Read the model definition and answer for the solid it produces. Units are mm, in the model's axes. Face numbers are marked on the shaded views. A direction names the side the tool comes from. Coordinates: 2 decimals unless noted, no trailing zeros. Loops run counter-clockwise (first coordinate to the right, second up) from the corner with the lowest first, then second, coordinate; pieces in that order, holes last. Notation, with made-up numbers: (-23, -12) -> (30, -12) arc R29 ccw to (30, 24) -> close; hole circle Ø9 at (62.25, -34). An arc over 180 degrees is marked (long way). Answer as CSV lines item,"result".
```python
from build123d import *

# Parameters (mm, degrees)
SKETCH_1_W          = 68.077724156
SKETCH_1_H          = 41.280670561
SKETCH_1_W_2        = 40
SKETCH_1_H_2        = 14
EXTRUDE_1_DEPTH     = 3
SKETCH_2_W          = 68.077724156
SKETCH_2_H          = 41.280670561
SKETCH_2_W_2        = 62.677724156
SKETCH_2_H_2        = 35.480670561
EXTRUDE_2_DEPTH     = 11.04005
SKETCH_3_W          = 7.040050383
SKETCH_3_H          = 11.280670561
CUT_EXTRUDE_1_DEPTH = 2.9
SKETCH_4_W          = 3
SKETCH_4_H          = 1.8
EXTRUDE_3_DEPTH     = 3
SKETCH_5_W          = 3
SKETCH_5_H          = 1.8
EXTRUDE_4_DEPTH     = 3
SKETCH_6_W          = 3
SKETCH_6_H          = 1.8
EXTRUDE_5_DEPTH     = 2
SKETCH_7_W          = 3
SKETCH_7_H          = 1.8
EXTRUDE_6_DEPTH     = 2
SKETCH_8_W          = 14
SKETCH_8_H          = 5
CUT_EXTRUDE_2_DEPTH = 2.9
SKETCH_9_W          = 1
SKETCH_9_H          = 15
CUT_EXTRUDE_3_DEPTH = 1
SKETCH_10_W         = 1.5
SKETCH_10_H         = 7
EXTRUDE_7_DEPTH     = 7
SKETCH_13_R         = 1.55
CUT_EXTRUDE_6_DEPTH = 2.5
SKETCH_14_W         = 4
SKETCH_14_H         = 1.5
EXTRUDE_8_DEPTH     = 11
SKETCH_15_W         = 4
SKETCH_15_H         = 1.5
EXTRUDE_9_DEPTH     = 10
CHAMFER_1_SIZE      = 3
FILLET_2_R          = 3
SKETCH_16_W         = 7
SKETCH_16_H         = 1.5
EXTRUDE_10_DEPTH    = 7
SKETCH_17_R         = 1.55
CUT_EXTRUDE_7_DEPTH = 2.5


with BuildPart() as part:
    # 草图1 → 凸台-拉伸1 (new body)
    with BuildSketch(Plane.XY):
        with Locations((18.003533133, 5.902999581)):
            Rectangle(SKETCH_1_W, SKETCH_1_H)
        with Locations((19, 6)):
            Rectangle(SKETCH_1_W_2, SKETCH_1_H_2, mode=Mode.SUBTRACT)
    extrude(amount=-EXTRUDE_1_DEPTH)

    # 草图2 → 凸台-拉伸2 (add)
    with BuildSketch(Plane(origin=(0, 0, -3), x_dir=(-1, 0, 0), z_dir=(0, 0, -1))):
        with Locations((-18.003533133, 5.902999581)):
            Rectangle(SKETCH_2_W, SKETCH_2_H)
        with Locations((-18.203533133, 5.902999581)):
            Rectangle(SKETCH_2_W_2, SKETCH_2_H_2, mode=Mode.SUBTRACT)
    extrude(amount=EXTRUDE_2_DEPTH)

    # 草图3 → 切除-拉伸1 (cut)
    with BuildSketch(Plane.ZY.offset(16.035328945)):
        with Locations((-10.520025192, 5.902999581)):
            Rectangle(SKETCH_3_W, SKETCH_3_H)
    extrude(amount=-CUT_EXTRUDE_1_DEPTH, mode=Mode.SUBTRACT)

    # 草图4 → 凸台-拉伸3 (add)
    with BuildSketch(Plane.XZ.offset(-23.643334861)):
        with Locations((48.042395211, -11.340050383)):
            Rectangle(SKETCH_4_W, SKETCH_4_H)
    extrude(amount=EXTRUDE_3_DEPTH)

    # 草图5 → 凸台-拉伸4 (add)
    with BuildSketch(Plane(origin=(0, -11.8373357, 0), x_dir=(1, 0, 0), z_dir=(0, 1, 0))):
        with Locations((48.042395211, 11.340050383)):
            Rectangle(SKETCH_5_W, SKETCH_5_H)
    extrude(amount=EXTRUDE_4_DEPTH)

    # 草图6 → 凸台-拉伸5 (add)
    with BuildSketch(Plane.XZ.offset(-23.643334861)):
        with Locations((-11.635328945, -11.340050383)):
            Rectangle(SKETCH_6_W, SKETCH_6_H)
    extrude(amount=EXTRUDE_5_DEPTH)

    # 草图7 → 凸台-拉伸6 (add)
    with BuildSketch(Plane(origin=(0, -11.8373357, 0), x_dir=(1, 0, 0), z_dir=(0, 1, 0))):
        with Locations((-11.635328945, 11.340050383)):
            Rectangle(SKETCH_7_W, SKETCH_7_H)
    extrude(amount=EXTRUDE_6_DEPTH)

    # 草图8 → 切除-拉伸2 (cut)
    with BuildSketch(Plane(origin=(0, 26.543334861, 0), x_dir=(1, 0, 0), z_dir=(0, 1, 0))):
        with Locations((39.042395211, 11.540050383)):
            Rectangle(SKETCH_8_W, SKETCH_8_H)
    extrude(amount=-CUT_EXTRUDE_2_DEPTH, mode=Mode.SUBTRACT)

    # 草图9 → 切除-拉伸3 (cut)
    with BuildSketch(Plane(origin=(52.042395211, 0, 0), x_dir=(0, 0, -1), z_dir=(1, 0, 0))):
        with Locations((13.540050383, -5.2373357)):
            Rectangle(SKETCH_9_W, SKETCH_9_H)
    extrude(amount=-CUT_EXTRUDE_3_DEPTH, mode=Mode.SUBTRACT)

    # 草图10 → 凸台-拉伸7 (add)
    with BuildSketch(Plane(origin=(52.042395211, 0, 0), x_dir=(0, 0, -1), z_dir=(1, 0, 0))):
        with Locations((13.290050383, 15.043334861)):
            Rectangle(SKETCH_10_W, SKETCH_10_H)
    extrude(amount=EXTRUDE_7_DEPTH)

    # 草图13 → 切除-拉伸6 (cut, through all)
    with BuildSketch(Plane.XY.offset(-12.540050383)):
        with Locations((56.542395211, 15.043334861)):
            Circle(SKETCH_13_R)
    extrude(amount=-CUT_EXTRUDE_6_DEPTH, mode=Mode.SUBTRACT)

    # 草图14 → 凸台-拉伸8 (add)
    with BuildSketch(Plane(origin=(0, 26.543334861, 0), x_dir=(1, 0, 0), z_dir=(0, 1, 0))):
        with Locations((0.964671055, 0.75)):
            Rectangle(SKETCH_14_W, SKETCH_14_H)
    extrude(amount=EXTRUDE_8_DEPTH)

    # 草图15 → 凸台-拉伸9 (add)
    with BuildSketch(Plane(origin=(0, 0, -1.5), x_dir=(-1, 0, 0), z_dir=(0, 0, -1))):
        with Locations((-0.964671055, 36.793334861)):
            Rectangle(SKETCH_15_W, SKETCH_15_H)
    extrude(amount=EXTRUDE_9_DEPTH)

    # 倒角1
    chamfer_1_edges = [part.edges().sort_by_distance(p)[0] for p in [
        (2.964671055, 26.543334861, -0.75),
        (-1.035328945, 26.543334861, -0.75),
    ]]
    chamfer(chamfer_1_edges, length=CHAMFER_1_SIZE)

    # 圆角2
    fillet_2_edges = [part.edges().sort_by_distance(p)[0] for p in [
        (0.964671055, 36.043334861, -1.5),
    ]]
    fillet(fillet_2_edges, radius=FILLET_2_R)

    # 草图16 → 凸台-拉伸10 (add)
    with BuildSketch(Plane.XZ.offset(14.7373357)):
        with Locations((17.464671055, -13.290050383)):
            Rectangle(SKETCH_16_W, SKETCH_16_H)
    extrude(amount=EXTRUDE_10_DEPTH)

    # 草图17 → 切除-拉伸7 (cut, through all)
    with BuildSketch(Plane.XY.offset(-12.540050383)):
        with Locations((17.464671055, -19.2373357)):
            Circle(SKETCH_17_R)
    extrude(amount=-CUT_EXTRUDE_7_DEPTH, mode=Mode.SUBTRACT)


solid = part.part
```
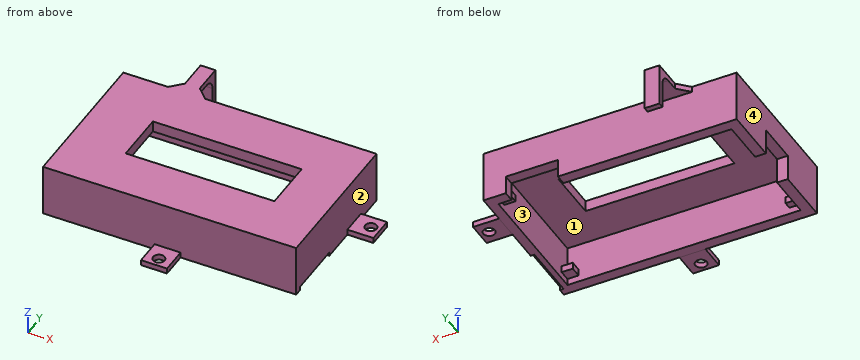
Q1. For the marked faces 3 and 4, determine the directions among +Z, -Z, +X, -X, +Y, -Y from which every point of the face is accessible in a straight line to the end or side of a thin tool.
Results:
face 3,"none"
face 4,"+Z, -Z, -X, +Y, -Y"
Q2. A cutting plane is placed at A-A, the plane x = 24.5. Write down the section's boundary in (y, z), and give its area (3 significant figures).
Results:
outline,"(-14.74, -14.04) -> (-11.84, -14.04) -> (-11.84, -3) -> (-1, -3) -> (-1, 0) -> (-14.74, 0) -> close; (13, -3) -> (23.64, -3) -> (23.64, -14.04) -> (26.54, -14.04) -> (26.54, 0) -> (13, 0) -> close"
area,"146 mm²"
Q3. Given pin 1 Ø3.5 at (x, y) = (47.5, -10.5) entering from -Z; pin 2 Ø7.5 at (x, y) = (18.5, -19) entering from +Z; pin 3 Ø4 at (y, z) = (34, -4) entering from -X; pin 4 Ø1.4 at (x, z) = (-12, -11.5) entering from +Y, each flat-ended and moving along its own axis, determine where each tip first touches the part or whether it passes through.
Results:
pin 1,"stops at z = -14.04"
pin 2,"stops at z = -12.54"
pin 3,"stops at x = -1.04"
pin 4,"stops at y = 26.54"
Q4. Find the intervals of material crossed by probe 1 along Y at (x, z) = (2, -5.25); probe 2 along Y at (x, z) = (7, -10.75); probe 3 along X at (y, z) = (21.5, -10.5), in increasing order. Write a range as [from, to].
Results:
probe 1,"y = [-14.74, -11.84], [23.64, 26.54], [36.04, 37.54]"
probe 2,"y = [-14.74, -11.84], [23.64, 26.54]"
probe 3,"x = [-16.04, -13.14], [46.54, 52.04]"
Q5. For a pull along Y with two mould halves and no side action, classify the marked faces 1 and 2 as pulls with the +Y half, pulls with the -Y half, needs draft (parallel to the pull), parting line crosses it, or undercut.
Results:
face 1,"undercut"
face 2,"needs draft"
Q6. A cutting plane is placed at B-B, the plane x = -5.5. Write down the section's boundary in (y, z).
Results:
outline,"(-14.74, -14.04) -> (-11.84, -14.04) -> (-11.84, -3) -> (23.64, -3) -> (23.64, -14.04) -> (26.54, -14.04) -> (26.54, 0) -> (-14.74, 0) -> close"
